Geometry: final body of the model. Coordinates: model frame, mm. Face numbers are marked on the shaded views. A direction names the side the tool comes from. Give positions to 0.01 mm unless a question says otherwise; leave off trailing zeros. Write each loop counter-clockwise with the first axis right and the second up, starting at its lowest first coordinate (ties: lowest second). Pieces come first, ordered by that corner, then holes.
Q1. Section B-B (x = 0.5). Return the cut outline in (y, z).
Q2. Line query: line 1 (Z direction, x = 2.5, y = 8.4); line 2 (Z direction, x = 2.5, y = 8); line 3 (Y direction, x = 2.4, z = 15.5). Output: solid intervals per line, ascending.
Q3. Pin query (flat end, axial travel): pin 1 Ø1.5 at (x, z) = (3.5, 5.5) entering from +Y; pin 2 Ø1 at (x, z) = (3, 16.5) entering from -Y; pin 3 Ø1.5 at (x, z) = (2, 13.5) entering from +Y. Return the tip coordinate at first contact, or that it passes through.
Q4. Reachability of the marked faces 1 and 2 from +Z, -Z, +X, -X, +Y, -Y: full face, straight path, thin tool, end or side. Return the list, or none.
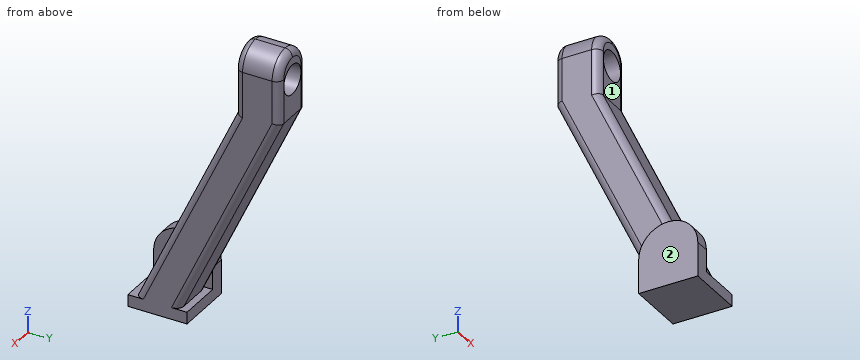
from build123d import *

# Parameters (mm, degrees)
F0_W      = 4
F0_H      = 4
F1_DEPTH  = 0.8
F4_DEPTH  = 1.5
F5_R      = 1
F6_DEPTH  = 10.2624610432
F7_R      = 1.49999
F8_R      = 0.49999
F10_DEPTH = 1


# Not quite as in the source:
# - a fillet or chamfer is up to 0.001 mm smaller than in the source, because OpenCascade refuses the exact size


with BuildPart() as f1:
    # F0 (on Top) → F1 (new body)
    with BuildSketch(Plane.XY):
        with Locations((2, 2)):
            Rectangle(F0_W, F0_H)
    extrude(amount=F1_DEPTH)

    # F3 (on offset) → F4 (join, symmetric)
    with BuildSketch(Plane.YZ.offset(2.5)):
        Polygon((0.5, 0.8), (3.5, 0.8), (10.2614610432, 15.3), (10.2614610432, 19.8), (7.2614610432, 19.8), (7.2614610432, 15.3), align=None)
    extrude(amount=F4_DEPTH, both=True)

    # F5 (on face) → F6 (cut, through all)
    with BuildSketch(Plane(origin=(0, 10.2614610432, 0), x_dir=(-1, 0, 0), z_dir=(0, 1, 0))):
        with Locations((-2.5, 17.8)):
            Circle(F5_R)
    extrude(amount=-F6_DEPTH, mode=Mode.SUBTRACT)

    # F7 (radius 1.5 in the source; OpenCascade refuses exactly that, so slightly less here)
    f7_edges = [f1.edges().sort_by_distance(p)[0] for p in [
        (1, 8.761461, 19.8),
        (4, 8.761461, 19.8),
    ]]
    fillet(f7_edges, radius=F7_R)

    # F8 (radius 0.5 in the source; OpenCascade refuses exactly that, so slightly less here)
    f8_edges = [f1.edges().sort_by_distance(p)[0] for p in [
        (1, 6.880731, 8.05),
        (1, 10.261461, 16.800005),
        (3.560663, 10.261461, 19.360663),
        (4, 6.880731, 8.05),
        (1, 3.880731, 8.05),
        (1, 7.261461, 16.800005),
        (4, 3.880731, 8.05),
    ]]
    fillet(f8_edges, radius=F8_R)

    # F9 (on face) → F10 (join)
    with BuildSketch(Plane(origin=(0, 0, 0), x_dir=(0, -1, 0), z_dir=(-1, 0, 0))):
        with BuildLine():
            Line((-4, 2.3), (-4, 0.8))
            Line((-4, 0.8), (0, 0.8))
            Line((0, 0.8), (0, 2.3))
            ThreePointArc((0, 2.3), (-0.5857864376, 3.7142135624), (-2, 4.3))
            ThreePointArc((-2, 4.3), (-3.4142135624, 3.7142135624), (-4, 2.3))
        make_face()
    extrude(amount=-F10_DEPTH)


solid = f1.part
Computed:
1. outline: (0, 0) - (4, 0) - (4, 2.3) arc R2 ccw to (0, 2.3) - close
2. line 1: z = 11.31 to 16.8, 18.8 to 19.8
2. line 2: z = 10.45 to 16.8, 18.8 to 19.8
2. line 3: y = 7.26 to 10.26
3. pin 1: stops at y = 6.04
3. pin 2: stops at y = 7.26
3. pin 3: stops at y = 9.77
4. face 1: +Z, +X, -X, -Y
4. face 2: +Z, -Z, -X, +Y, -Y
